Geometry check sheet. Reference: the model listing, model coordinates, mm. Face numbers are marked on the shaded views. A direction names the side the tool comes from. Give positions to 0.01 mm unless a question says otherwise; leave off trailing zeros. Write each loop counter-clockwise with the first axis right and the second up, starting at its lowest first coordinate (ties: lowest second). Pieces come first, ordered by that corner, then holes. Notation, with made-up numbers: (55, -18) - (73, -18) arc R29 ccw to (73, 14) - close; hole circle Ø2 at (73, 42). An arc over 180 degrees is marked (long way). Use a Markdown table: item, result.
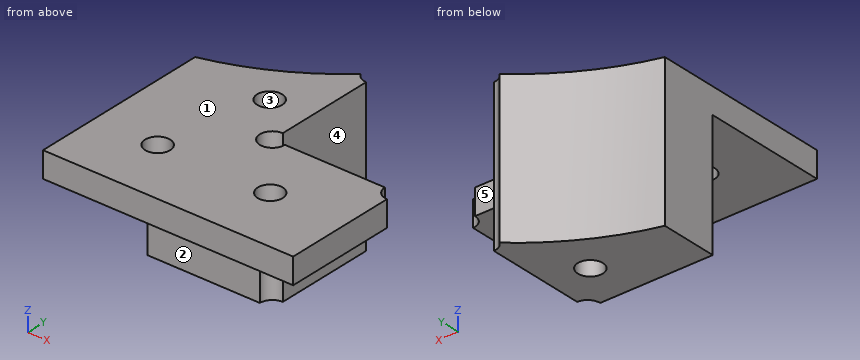
```python
from build123d import *

# Parameters (mm, degrees)
SKETCH_1_W          = 20
SKETCH_1_H          = 20
SKETCH_1_R          = 2
EXTRUDE_1_DEPTH     = 4.1
SKETCH_2_W          = 20
SKETCH_2_H          = 20
EXTRUDE_2_DEPTH     = 24.1
CUT_EXTRUDE_1_DEPTH = 40.759401404
SKETCH_4_R          = 2
CUT_EXTRUDE_2_DEPTH = 40.759401404
SKETCH_5_W          = 4.1
SKETCH_5_H          = 20
EXTRUDE_3_DEPTH     = 20
SKETCH_7_R          = 2
CUT_EXTRUDE_3_DEPTH = 49.793544655


with BuildPart() as part:
    # 草图1 → 凸台-拉伸1 (new body)
    with BuildSketch(Plane.XY):
        Rectangle(SKETCH_1_W, SKETCH_1_H)
        Circle(SKETCH_1_R, mode=Mode.SUBTRACT)
    extrude(amount=EXTRUDE_1_DEPTH)

    # 草图2 → 凸台-拉伸2 (add)
    with BuildSketch(Plane.XY.offset(4.1)):
        with Locations((0, 20)):
            Rectangle(SKETCH_2_W, SKETCH_2_H)
    extrude(amount=-EXTRUDE_2_DEPTH)

    # 草图3 → 切除-拉伸1 (cut, through all)
    with BuildSketch(Plane.XY.offset(4.1)):
        with BuildLine():
            Line((-10, 30), (9.2059994, 30))
            ThreePointArc((9.2059994, 30), (0.308275872, 23.337476197), (-10, 19.178371007))
            Line((-10, 19.178371007), (-10, 30))
        make_face()
    extrude(amount=-CUT_EXTRUDE_1_DEPTH, mode=Mode.SUBTRACT)

    # 草图4 → 切除-拉伸2 (cut, through all)
    with BuildSketch(Plane.XY.offset(4.1)):
        with Locations((3.589185504, 17.178371007)):
            Circle(SKETCH_4_R)
    extrude(amount=-CUT_EXTRUDE_2_DEPTH, mode=Mode.SUBTRACT)

    # 草图5 → 凸台-拉伸3 (add)
    with BuildSketch(Plane(origin=(10, 0, 0), x_dir=(0, 0, -1), z_dir=(1, 0, 0))):
        with Locations((-2.05, 0)):
            Rectangle(SKETCH_5_W, SKETCH_5_H)
    extrude(amount=EXTRUDE_3_DEPTH)

    # 草图7 → 切除-拉伸3 (cut, through all)
    with BuildSketch(Plane.XY.offset(4.1)):
        with Locations((10, 10)):
            Circle(SKETCH_7_R)
        with Locations((10, 30)):
            Circle(SKETCH_7_R)
        with Locations((30, 10)):
            Circle(SKETCH_7_R)
        with Locations((18, 0)):
            Circle(SKETCH_7_R)
    extrude(amount=-CUT_EXTRUDE_3_DEPTH, mode=Mode.SUBTRACT)


solid = part.part
```
1) Material ranges on L1, parallel to Y at x = 18, z = 1.95; L2, parallel to Z at x = 28, y = -2; L3, parallel to X at y = 15, z = -15.75, recorded low to high. Write a range as from..to.
Working result:
| item | result |
|---|---|
| L1 | y = -10..-2, 2..10 |
| L2 | z = 0..4.1 |
| L3 | x = -10..10 |
2) Mould release check, pull along X, two halves, no side actions. Record for the marked faces 3, 4 and 5: pulls with the +X half, pulls with the -X half, needs draft (parallel to the pull), parting line crosses it, or undercut.
Working result:
| item | result |
|---|---|
| face 3 | undercut |
| face 4 | pulls with the +X half |
| face 5 | needs draft |
3) Section check A-A on x = 18. Record the boundary of the cut face in (y, z), then the cut area to 3 significant figures.
Working result:
| item | result |
|---|---|
| outline | (-10, 0) - (-2, 0) - (-2, 4.1) - (-10, 4.1) - close; (2, 0) - (10, 0) - (10, 4.1) - (2, 4.1) - close |
| area | 65.6 mm² |
4) Section check C-C on z = -15.75. Record the boundary of the cut face in (x, y), then the cut area to 3 significant figures.
Working result:
| item | result |
|---|---|
| outline | (-10, 10) - (8, 10) arc R2 cw to (10, 12) - (10, 28) arc R2 cw to (8.23, 29.08) arc R43 cw to (-10, 19.18) - close; hole circle Ø4 at (3.59, 17.18) |
| area | 257 mm² |
5) Depth check by flat-ended pin: P1, Ø1.5, axis at x = 9.5, z = -6.5, coming from the +Y side; P2, Ø4.5, axis at x = 24, z = 1.5, coming from the +Y side; P3, Ø5, axis at y = 23, z = -9.5, coming from the +X side. Enter the tip coordinate at first touch or a pass-through.
Working result:
| item | result |
|---|---|
| P1 | stops at y = 28.44 |
| P2 | stops at y = 10 |
| P3 | stops at x = 10 |
6) Section check D-D on y = 16. Record the boundary of the cut face in (x, z), then the cut area to 3 significant figures.
Working result:
| item | result |
|---|---|
| outline | (-10, -20) - (1.97, -20) - (1.97, 4.1) - (-10, 4.1) - close; (5.21, -20) - (10, -20) - (10, 4.1) - (5.21, 4.1) - close |
| area | 404 mm² |
7) Set-up check for the marked faces 1 and 2: record each of +Z, -Z, +X, -X, +Y, -Y from which the full face is reachable in a straight line by a thin tool's end or side.
Working result:
| item | result |
|---|---|
| face 1 | +Z, +X, -X, +Y, -Y |
| face 2 | -Z, +X, -X, -Y |
8) Section check B-B on y = 0. Record the boundary of the cut face in (x, z).
Working result:
| item | result |
|---|---|
| outline | (-10, 0) - (-2, 0) - (-2, 4.1) - (-10, 4.1) - close; (2, 0) - (16, 0) - (16, 4.1) - (2, 4.1) - close; (20, 0) - (30, 0) - (30, 4.1) - (20, 4.1) - close |
